from build123d import *

# Parameters (mm, degrees)
SKETCH1_W               = 95
SKETCH1_H               = 54
SKETCH1_W_2             = 92
SKETCH1_H_2             = 51
BOSS_EXTRUDE1_DEPTH     = 20
SKETCH2_W               = 2
SKETCH2_H               = 2
BOSS_EXTRUDE2_DEPTH     = 20
FILLET1_R               = 1
CUT_EXTRUDE1_DEPTH      = 75.647504982
CUT_EXTRUDE1_DEPTH_BACK = 75.647504982
SKETCH3_W               = 14
SKETCH3_H               = 2
FILLET2_R               = 1
FILLET3_R               = 0.5


with BuildPart() as part:
    # Sketch1 → Boss-Extrude1 (new body)
    with BuildSketch(Plane.XY):
        Rectangle(SKETCH1_W, SKETCH1_H)
        Rectangle(SKETCH1_W_2, SKETCH1_H_2, mode=Mode.SUBTRACT)
    extrude(amount=BOSS_EXTRUDE1_DEPTH)

    # Sketch2 → Boss-Extrude2 (add)
    with BuildSketch(Plane(origin=(0, 0, 0), x_dir=(-1, 0, 0), z_dir=(0, 0, -1))):
        with Locations((22, 24.5)):
            Rectangle(SKETCH2_W, SKETCH2_H)
        with Locations((-38, 24.5)):
            Rectangle(SKETCH2_W, SKETCH2_H)
        with Locations((38, 24.5)):
            Rectangle(SKETCH2_W, SKETCH2_H)
        with Locations((-22, 24.5)):
            Rectangle(SKETCH2_W, SKETCH2_H)
        with Locations((38, -24.5)):
            Rectangle(SKETCH2_W, SKETCH2_H)
        with Locations((22, -24.5)):
            Rectangle(SKETCH2_W, SKETCH2_H)
        with Locations((-22, -24.5)):
            Rectangle(SKETCH2_W, SKETCH2_H)
        with Locations((-38, -24.5)):
            Rectangle(SKETCH2_W, SKETCH2_H)
    extrude(amount=-BOSS_EXTRUDE2_DEPTH)

    # Fillet1
    fillet1_edges = [part.edges().sort_by_distance(p)[0] for p in [
        (-46, -25.5, 10),
        (-46, 25.5, 10),
        (46, -25.5, 10),
        (39, -25.5, 10),
        (39, -23.5, 10),
        (21, -23.5, 10),
        (21, -25.5, 10),
        (-21, -25.5, 10),
        (-21, -23.5, 10),
        (-39, -23.5, 10),
        (-39, -25.5, 10),
        (-39, 25.5, 10),
        (-39, 23.5, 10),
        (-21, 23.5, 10),
        (-21, 25.5, 10),
        (21, 25.5, 10),
        (21, 23.5, 10),
        (39, 23.5, 10),
        (39, 25.5, 10),
        (46, 25.5, 10),
    ]]
    fillet(fillet1_edges, radius=FILLET1_R - 0.0001)  # a hair under: the kernel refuses the full size

    # Sketch3 → Cut-Extrude1 (cut, two sides: drawn at the far end of the back side and taken through both)
    with BuildSketch(Plane.XZ.offset(27).offset(-CUT_EXTRUDE1_DEPTH_BACK)):
        with Locations((-30, 10)):
            Rectangle(SKETCH3_W, SKETCH3_H)
        with Locations((30, 10)):
            Rectangle(SKETCH3_W, SKETCH3_H)
        with Locations((30, 19)):
            Rectangle(SKETCH3_W, SKETCH3_H)
        with Locations((-30, 19)):
            Rectangle(SKETCH3_W, SKETCH3_H)
    extrude(amount=CUT_EXTRUDE1_DEPTH + CUT_EXTRUDE1_DEPTH_BACK, mode=Mode.SUBTRACT)

    # Fillet2
    fillet2_edges = [part.edges().sort_by_distance(p)[0] for p in [
        (-30, -25.5, 18),
        (-30, 25.5, 18),
        (30, -25.5, 18),
        (30, 25.5, 18),
    ]]
    fillet(fillet2_edges, radius=FILLET2_R)

    # Fillet3
    fillet3_edges = [part.edges().sort_by_distance(p)[0] for p in [
        (30, -25.5, 9),
        (30, 25.5, 9),
        (30, -25.5, 11),
        (30, 25.5, 11),
        (-30, -25.5, 11),
        (-30, 25.5, 11),
        (-30, -25.5, 9),
        (-30, 25.5, 9),
    ]]
    fillet(fillet3_edges, radius=FILLET3_R)


solid = part.part
Geometry check sheet. Reference: the model listing, model coordinates, mm. A direction names the side the tool comes from. Round coordinates to 2 decimals unless told otherwise and drop trailing zeros. Write each loop counter-clockwise with the first axis right and the second up, starting at its lowest first coordinate (ties: lowest second). Pieces come first, ordered by that corner, then holes.
Item 1: Access from +Z, -Z, +X, -X, +Y, -Y to the whole of each face (thin tool, end or side, straight path). Record for faces 4 (the face through (42, -25.5, 10)), 5 (the face through (0, 26, 0)).
Determined:
face 4: +Z, -Z
face 5: -Z, +X, -X, +Y, -Y
Item 2: Section check A-A (x = 34). Record the boundary of the cut face in (y, z).
Determined:
outline: (-27, 0) - (-25.5, 0) - (-25.5, 8.5) arc R0.5 ccw to (-26, 9) - (-27, 9) - close; (-27, 11) - (-26, 11) arc R0.5 ccw to (-25.5, 11.5) - (-25.5, 17) arc R1 ccw to (-26.5, 18) - (-27, 18) - close; (25.5, 0) - (27, 0) - (27, 9) - (26, 9) arc R0.5 ccw to (25.5, 8.5) - close; (25.5, 11.5) arc R0.5 ccw to (26, 11) - (27, 11) - (27, 18) - (26.5, 18) arc R1 ccw to (25.5, 17) - close
Item 3: Material ranges on line 1 along Y through (x, z) = (14, 4); line 2 along X through (y, z) = (5, 16); line 3 along Y through (x, z) = (37.5, 9.5), recorded low to high.
Determined:
line 1: y = -27 to -25.5, 25.5 to 27
line 2: x = -47.5 to -46, 46 to 47.5
line 3: y = -27 to -23.5, 23.5 to 27
Item 4: Section check C-C (x = -8). Record the boundary of the cut face in (y, z).
Determined:
outline: (-27, 0) - (-25.5, 0) - (-25.5, 20) - (-27, 20) - close; (25.5, 0) - (27, 0) - (27, 20) - (25.5, 20) - close
Item 5: Section check B-B (y = 11). Record the boundary of the cut face in (x, z).
Determined:
outline: (-47.5, 0) - (-46, 0) - (-46, 20) - (-47.5, 20) - close; (46, 0) - (47.5, 0) - (47.5, 20) - (46, 20) - close
Item 6: Go/stop test with a flat-tipped pin: pin 1 Ø0.8 at (x, y) = (-27, 26.5) entering from -Z. Record where the tip stops, or that it passes through.
Determined:
pin 1: stops at z = 0
Item 7: Mould release check, pull along X, two halves, no side actions. Record for faces 1 (the face through (-1, 27, 10)), 2 (the face through (46, 0, 10)), 3 (the face through (-47.5, 0, 10)): +X half, -X half, draft (parallel to the pull), parting line (faces both ways), or undercut.
Determined:
face 1: draft
face 2: undercut
face 3: -X half
